For this review, take the finished solid that the model builds, in its own axes (mm). Face numbers are marked on the shaded views. A direction names the side the tool comes from. Coordinates: 2 decimals unless noted, no trailing zeros. Write each loop counter-clockwise with the first axis right and the second up, starting at its lowest first coordinate (ties: lowest second). Pieces come first, ordered by that corner, then holes.
1) For the marked faces 4, 5 and 6, list the 3-axis set-ups (+Z, -Z, +X, -X, +Y, -Y) from which the entire face can be reached by the end or side of a thin tool; tool diameter is ignored.
2) To check wall thickness, follow line 1 along X through (y, z) = (126, 18.25); line 2 along Y through (x, z) = (56.5, 7.5); line 3 along Y through (x, z) = (-30, 11). State the ranges of each line that lie inside material, in increasing order.
3) We need section B-B on x = 0. Write out the cut boundary in (y, z).
4) We need section A-A on y = 0. Write out the cut boundary in (x, z), then the cut area to 3 significant figures.
5) Insertion check: P1, Ø5, axis at x = -8.5, z = 7, coming from the +Y side; P2, Ø4, axis at y = -78.5, z = 7.5, coming from the +X side; P3, Ø9.5, axis at x = 53.07, y = 133.57, coming from the -Z side; P4, Ø1, axis at y = 110, z = 4, coming from the +X side. Each pin has a flat end and moves straight along its axis. Give the tip position at first contact, or say it passes through.
6) Mouldability with a two-part tool opening along X and no side actions: class the marked faces 1, 2 and 3 as pulls with the +X half, pulls with the -X half, needs draft (parallel to the pull), parting line crosses it, or undercut.
from build123d import *

# Parameters (mm, degrees)
BOSS_EXTRUDE1_DEPTH             = 23
FILLET2_R                       = 50.8
SKETCH2_R                       = 40.05
CUT_EXTRUDE1_DEPTH              = 16
SKETCH5_R                       = 36.83
CUT_EXTRUDE2_DEPTH              = 25.4
FILLET5_R                       = 1
FILLET6_R                       = 1
CBORE_FOR_M10_SHCS7_D           = 10.5
CBORE_FOR_M10_SHCS7_CBORE_D     = 18
CBORE_FOR_M10_SHCS7_CBORE_DEPTH = 12
F_10_0MM_DOWEL_HOLE3_D          = 10
F_10_0MM_DOWEL_HOLE3_DEPTH      = 10
F_10_0MM_DOWEL_HOLE3_TIP        = 3.004303095
TAP_DRILL_FOR_3_8_16_TAP1_D     = 7.9375


with BuildPart() as part:
    # Sketch1 → Boss-Extrude1 (new body)
    with BuildSketch(Plane.XY):
        with BuildLine():
            Line((84.221105008, -163.490124242), (2.699306526, -136.831626991))
            Line((2.699306526, -136.831626991), (-67.458438584, -162.730244564))
            ThreePointArc((-67.458438584, -162.730244564), (-75.680634631, -163.297391653), (-82.910842941, -159.341351783))
            Line((-82.910842941, -159.341351783), (-126.914053579, -115.336397895))
            ThreePointArc((-126.914053579, -115.336397895), (-130.093640928, -110.577690662), (-131.210211433, -104.964461595))
            Line((-131.210211433, -104.964461595), (-131.213297338, 125.035476514))
            ThreePointArc((-131.213297338, 125.035476514), (-126.350161673, 135.869915187), (-115.02264263, 139.436771249))
            Line((-115.02264263, 139.436771249), (-20.796830867, 128.37488637))
            Line((-20.796830867, 128.37488637), (49.24312976, 147.55277548))
            ThreePointArc((49.24312976, 147.55277548), (58.421803723, 147.044752766), (65.450410839, 141.119820294))
            Line((65.450410839, 141.119820294), (107.841002341, 71.642808501))
            ThreePointArc((107.841002341, 71.642808501), (117.701476238, 53.952608996), (124.683759391, 34.941564155))
            Line((124.683759391, 34.941564155), (145.845410308, -40.455794779))
            ThreePointArc((145.845410308, -40.455794779), (145.61886709, -49.11646402), (140.544799405, -56.138739339))
            Line((140.544799405, -56.138739339), (109.149264581, -79.773969292))
            Line((109.149264581, -79.773969292), (103.401152517, -150.732337669))
            ThreePointArc((103.401152517, -150.732337669), (96.90432541, -161.761540655), (84.221105008, -163.490124242))
        make_face()
    extrude(amount=BOSS_EXTRUDE1_DEPTH)

    # Fillet2
    fillet2_edges = [part.edges().sort_by_distance(p)[0] for p in [
        (109.149264581, -79.773969292, 11.5),
        (2.699306526, -136.831626991, 11.5),
        (-20.796830867, 128.37488637, 11.5),
    ]]
    fillet(fillet2_edges, radius=FILLET2_R)

    # Sketch2 → Cut-Extrude1 (cut)
    with BuildSketch(Plane(origin=(0, 0, 23), x_dir=(-1, 0, 0), z_dir=(0, 0, -1))):
        Circle(SKETCH2_R)
    extrude(amount=CUT_EXTRUDE1_DEPTH, mode=Mode.SUBTRACT)

    # Sketch5 → Cut-Extrude2 (cut)
    with BuildSketch(Plane(origin=(0, 0, 23), x_dir=(-1, 0, 0), z_dir=(0, 0, -1))):
        Circle(SKETCH5_R)
    extrude(amount=CUT_EXTRUDE2_DEPTH, mode=Mode.SUBTRACT)

    # Fillet5
    fillet5_edges = [part.edges().sort_by_distance(p)[0] for p in [
        (40.05, 0, 23),
    ]]
    fillet(fillet5_edges, radius=FILLET5_R)

    # Fillet6
    fillet6_edges = [part.edges().sort_by_distance(p)[0] for p in [
        (40.05, 0, 7),
    ]]
    fillet(fillet6_edges, radius=FILLET6_R)

    # CBORE for M10 SHCS7 (through all)
    with Locations(Plane.XY.offset(23)):
        with Locations((-116.713297339, 125.03567106), (-116.541509562, -104.964264785), (-72.538298924, -148.969218673), (53.072470058, 133.567563544), (131.722431635, -44.419667636), (88.780343848, -149.547952394)):
            CounterBoreHole(CBORE_FOR_M10_SHCS7_D / 2, CBORE_FOR_M10_SHCS7_CBORE_D / 2, CBORE_FOR_M10_SHCS7_CBORE_DEPTH)

    # Ø10.0mm Dowel Hole3
    with Locations(Plane(origin=(0, 0, 0), x_dir=(-1, 0, 0), z_dir=(0, 0, -1))):
        with Locations((76.55340813, 103.753913834), (-59.102558089, -114.980445858)):
            Hole(F_10_0MM_DOWEL_HOLE3_D / 2, depth=F_10_0MM_DOWEL_HOLE3_DEPTH)
            with Locations((0, 0, -(F_10_0MM_DOWEL_HOLE3_DEPTH + F_10_0MM_DOWEL_HOLE3_TIP / 2))):  # 118° drill point
                Cone(0, F_10_0MM_DOWEL_HOLE3_D / 2, F_10_0MM_DOWEL_HOLE3_TIP, mode=Mode.SUBTRACT)

    # Tap Drill for 3/8-16 Tap1 (through all)
    with Locations(Plane(origin=(75.504350667, 75.417116381, 23), x_dir=(1, 0, 0), z_dir=(0, 0, 1))):
        with Locations((0, 0), (-150.921467048, 0.087234286), (-151.008701334, -150.834232762), (-0.087234286, -150.921467048)):
            Hole(TAP_DRILL_FOR_3_8_16_TAP1_D / 2)


solid = part.part
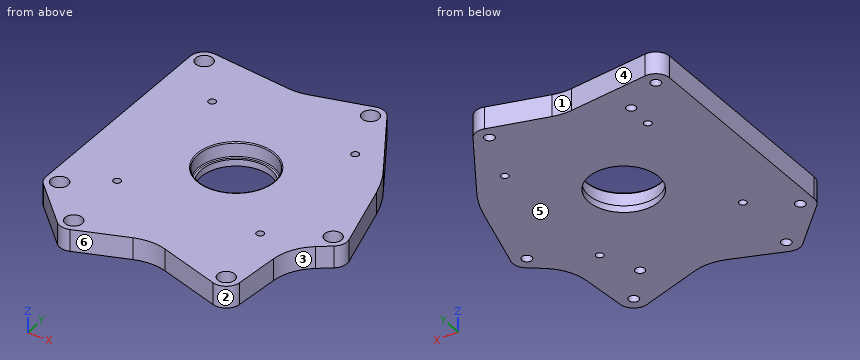
Result:
1. face 4: +Z, -Z, +Y
1. face 5: -Z, +X, -X, +Y, -Y
1. face 6: +Z, -Z, -Y
2. line 1: x = -131.18 to -125.66, -107.77 to 48.2, 57.94 to 74.68
2. line 2: y = -154.43 to -119.25, -110.71 to 129.59, 137.54 to 147.66
2. line 3: y = -148.9 to -26.53, 26.53 to 129.46
3. outline: (-139.94, 0) - (-36.83, 0) - (-36.83, 7) - (-39.05, 7) arc R1 cw to (-40.05, 8) - (-40.05, 22) arc R1 ccw to (-41.05, 23) - (-139.94, 23) - close; (36.83, 0) - (134.07, 0) - (134.07, 23) - (41.05, 23) arc R1 ccw to (40.05, 22) - (40.05, 8) arc R1 cw to (39.05, 7) - (36.83, 7) - close
4. outline: (-131.21, 0) - (-36.83, 0) - (-36.83, 7) - (-39.05, 7) arc R1 cw to (-40.05, 8) - (-40.05, 22) arc R1 ccw to (-41.05, 23) - (-131.21, 23) - close; (36.83, 0) - (134.49, 0) - (134.49, 23) - (41.05, 23) arc R1 ccw to (40.05, 22) - (40.05, 8) arc R1 cw to (39.05, 7) - (36.83, 7) - close
4. area: 4,310 mm2
5. P1: stops at y = 132.43
5. P2: stops at x = 117.04
5. P3: passes through
5. P4: stops at x = 84.74
6. face 1: undercut
6. face 2: parting line crosses it
6. face 3: pulls with the +X half
